The figure shows three views and two pictorial views of one solid part (mm, origin at its lowest corner). Answer the questions. A direction names the side the tool comes from. Round coordinates to 2 decimals unless told otherwise and drop trailing zeros. Order: outer loops, then holes, each group sorted by start corner. A loop starts at its lowest first (then second) coordinate and runs counter-clockwise, first axis right, second up. Notation, with made-up numbers: (50.25, 60) - (98.25, 60) arc R24 cw to (98.25, 71) - close; hole circle Ø8 at (1.5, 36.5). An arc over 180 degrees is marked (long way). Use CSV: the item, a comma, the result in double quotes.
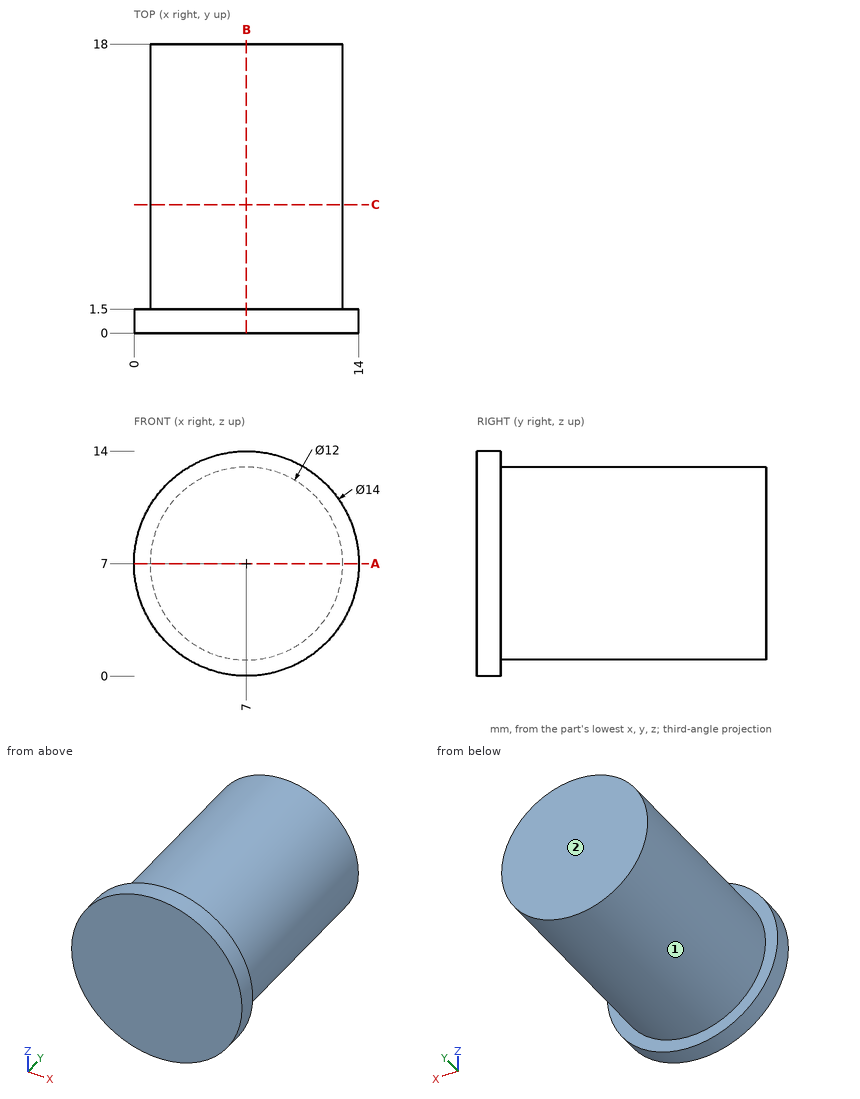
(1) Find section C-C (y = 8). Determine the outline of the cut face in (x, z).
Findings below:
outline,"circle Ø12 at (7, 7)"
(2) For the marked faces 1 and 2, determine the directions among +Z, -Z, +X, -X, +Y, -Y from which every point of the face is accessible in a straight line to the end or side of a thin tool.
Findings below:
face 1,"+Y"
face 2,"+Z, -Z, +X, -X, +Y"
(3) Find section A-A (z = 7). Determine the outline of the cut face in (x, y).
Findings below:
outline,"(0, 0) - (14, 0) - (14, 1.5) - (13, 1.5) - (13, 18) - (1, 18) - (1, 1.5) - (0, 1.5) - close"
(4) Find the intervals of material crossed by L1, parallel to Y at x = 0.75, z = 8.5; L2, parallel to X at y = 16.25, z = 7.25; L3, parallel to Z at x = 4, y = 14.25, in increasing order. Write a range as from..to.
Findings below:
L1,"y = 0..1.5"
L2,"x = 1.01..12.99"
L3,"z = 1.8..12.2"
(5) Each of these flat-tipped pins is pushed along its axis until it touches: pin 1 (2 mm diameter, centred on y = 9.5, z = 8, fed in from +X); pin 2 (3 mm diameter, centred on y = 13.5, z = 3.5, fed in from +X); pin 3 (2 mm diameter, centred on y = 13, z = 9.5, fed in from +X). Where does it stop, or does it pass through?
Findings below:
pin 1,"stops at x = 13"
pin 2,"stops at x = 12.66"
pin 3,"stops at x = 12.81"
(6) Find section B-B (x = 7). Determine the outline of the cut face in (y, z), and give its area (3 significant figures).
Findings below:
outline,"(0, 0) - (1.5, 0) - (1.5, 1) - (18, 1) - (18, 13) - (1.5, 13) - (1.5, 14) - (0, 14) - close"
area,"219 mm²"
